Check sheet for the modelled part. Datum: model origin and axes. Units: mm. A direction names the side the tool comes from. Round coordinates to 2 decimals unless told otherwise and drop trailing zeros. Order: outer loops, then holes, each group sorted by start corner. A loop starts at its lowest first (then second) coordinate and runs counter-clockwise, first axis right, second up.
(1) Sectioned sample at C-C, the plane y = 2. Enter the section's corners in (x, z).
(2) Tool access check on faces 5 (the flat face through (-2.36, 0.01, 0.15)), 6 (the flat face through (-6, -5.39, 0.15)), 7 (the flat face through (-6.6, -2, 1)). Record the directions out of +Z, -Z, +X, -X, +Y, -Y that give a thin tool (end or side, any length) a straight path to the whole face; none if there is none.
(3) Thickness scan on probe 1 along Y at (x, z) = (0, 1.1); probe 2 along X at (y, z) = (14.75, 1.65); probe 3 along X at (y, z) = (4, 1.3). Record the ranges inside material, lowest first.
(4) Sectioned sample at B-B, the plane z = 0.95. Enter the section's corners in (x, y).
(5) Mould release check, pull along X, two halves, no side actions. Record for faces 1 (the flat face through (2.166, 0.142, 1.187)), 2 (the flat face through (-6, 4, 1)), 3 (the flat face through (-5, -6, 1)), 4 (the flat face through (6, 3, 1)): released by +X, released by -X, zero draft, split by the parting line, or undercut.
(6) Depth check by flat-ended pin: pin 1 (0.5 mm diameter, centred on y = 2.5, z = 1.5, fed in from +X); pin 2 (0.9 mm diameter, centred on y = -1.5, z = 1.5, fed in from +X); pin 3 (0.5 mm diameter, centred on y = 3.5, z = 1.5, fed in from -X); pin 4 (5.5 mm diameter, centred on x = 0, y = 12, fed in from +Z). Enter the tip coordinate at first touch or a pass-through.
(7) Sectioned sample at A-A, the plane x = 0. Enter the section's corners in (y, z).
```python
from build123d import *

# Parameters (mm, degrees)
SKETCH1_R           = 3.399254874
BOSS_EXTRUDE1_DEPTH = 2.1
CHAMFER1_SIZE       = 1
CHAMFER2_SIZE       = 0.3


with BuildPart() as part:
    # Sketch1 → Boss-Extrude1 (new body)
    with BuildSketch(Plane.XY):
        with BuildLine():
            Line((6, 6), (12, 6))
            ThreePointArc((12, 6), (0, 18), (-12, 6))
            Line((-12, 6), (-6, 6))
            Line((-6, 6), (-6, 1))
            Line((-6, 1), (-6.6, 1))
            Line((-6.6, 1), (-6.6, -6))
            Line((-6.6, -6), (-6, -6))
            Line((-6, -6), (-4, -6))
            Line((-4, -6), (-0.383283535, 6.114427845))
            ThreePointArc((-0.383283535, 6.114427845), (0, 6.4), (0.383283535, 6.114427845))
            Line((0.383283535, 6.114427845), (4, -6))
            Line((4, -6), (6, -6))
            Line((6, -6), (6.6, -6))
            Line((6.6, -6), (6.6, 1))
            Line((6.6, 1), (6, 1))
            Line((6, 1), (6, 6))
        make_face()
        with Locations((0, 12)):
            Circle(SKETCH1_R, mode=Mode.SUBTRACT)
    extrude(amount=BOSS_EXTRUDE1_DEPTH)

    # Chamfer1
    chamfer1_edges = [part.edges().sort_by_distance(p)[0] for p in [
        (-6.6, -6, 1.05),
        (6.6, -6, 1.05),
    ]]
    chamfer(chamfer1_edges, length=CHAMFER1_SIZE)

    # Chamfer2
    chamfer2_edges = [part.edges().sort_by_distance(p)[0] for p in [
        (2.191641768, 0.057213923, 0),
        (0, 6.4, 0),
        (-2.191641768, 0.057213923, 0),
        (-6.6, -2, 0),
        (-6.3, 1, 0),
        (-6, 3.5, 0),
        (-9, 6, 0),
        (0, 18, 0),
        (9, 6, 0),
        (6, 3.5, 0),
        (6.3, 1, 0),
        (4.8, -6, 0),
        (-3.399254874, 12, 0),
        (6.6, -2, 0),
        (-4.8, -6, 0),
        (-6.1, -5.5, 0),
        (6.1, -5.5, 0),
    ]]
    chamfer(chamfer2_edges, length=CHAMFER2_SIZE)


solid = part.part
```
Derived:
1. outline: (-6, 0.3) - (-5.7, 0) - (-1.92, 0) - (-1.61, 0.3) - (-1.61, 2.1) - (-6, 2.1) - close; (1.61, 0.3) - (1.92, 0) - (5.7, 0) - (6, 0.3) - (6, 2.1) - (1.61, 2.1) - close
2. face 5: -Z, -Y
2. face 6: -Z, -X, -Y
2. face 7: +Z, -Z, -X, -Y
3. probe 1: y = 6.4 to 8.6, 15.4 to 18
3. probe 2: x = -8.21 to -2, 2 to 8.21
3. probe 3: x = -6 to -1.01, 1.01 to 6
4. outline: (-12, 6) - (-6, 6) - (-6, 1) - (-6.6, 1) - (-6.6, -5) - (-5.6, -6) - (-4, -6) - (-0.38, 6.11) arc R0.4 cw to (0.38, 6.11) - (4, -6) - (5.6, -6) - (6.6, -5) - (6.6, 1) - (6, 1) - (6, 6) - (12, 6) arc R12 ccw to start; hole circle Ø6.8 at (0, 12)
5. face 1: undercut
5. face 2: released by -X
5. face 3: zero draft
5. face 4: released by +X
6. pin 1: stops at x = 6
6. pin 2: stops at x = 6.6
6. pin 3: stops at x = -6
6. pin 4: passes through
7. outline: (6.4, 0.3) - (6.7, 0) - (8.3, 0) - (8.6, 0.3) - (8.6, 2.1) - (6.4, 2.1) - close; (15.4, 0.3) - (15.7, 0) - (17.7, 0) - (18, 0.3) - (18, 2.1) - (15.4, 2.1) - close
